```python
from build123d import *

# Parameters (mm, degrees)
SKETCH_1_R             = 6.25
SM_BASE_FLANGE_1_DEPTH = 6
OTHER_START            = 4.8
OTHER_1_OUTLINE_W      = 4.4
OTHER_1_OUTLINE_H      = 6
OTHER_1_DEPTH          = 20.4
OTHER_START_2          = 41.159902189
OTHER_1_2_OUTLINE_W    = 4.4
OTHER_1_2_OUTLINE_H    = 6
OTHER_1_2_DEPTH        = 20.4
OTHER_START_3          = 77.519804378
OTHER_1_3_OUTLINE_W    = 4.4
OTHER_1_3_OUTLINE_H    = 6
OTHER_1_3_DEPTH        = 20.4


# Read off the part's stored shape, not the designer's step: Выступы и прорези-Прорезь1
# Sheet-metal steps are written as plain solids
with BuildPart() as part:
    # Sketch 1 → Базовая кромка1 (new body)
    with BuildSketch(Plane.XY):
        with BuildLine():
            Line((0, 0), (0, -23))
            Line((0, -23), (92.230562732, -113.222677357))
            ThreePointArc((92.230562732, -113.222677357), (113.643192103, -112.780058395), (112.786839702, -91.379982025))
            ThreePointArc((112.786839702, -91.379982025), (92.360596545, -22.078545096), (144.700960487, 27.725138224))
            ThreePointArc((144.700960487, 27.725138224), (156.538037696, 42.016473572), (145.424946819, 56.877761338))
            ThreePointArc((145.424946819, 56.877761338), (102.719804378, 62.5), (60.014661936, 56.877761338))
            ThreePointArc((60.014661936, 56.877761338), (56.414969483, 55.389643277), (53.319804477, 53.024852653))
            Line((53.319804477, 53.024852653), (0, 0))
        make_face()
        with Locations((102.719804378, -102.5)):
            Circle(SKETCH_1_R, mode=Mode.SUBTRACT)
        with Locations((141.542661143, 42.388873943)):
            Circle(SKETCH_1_R, mode=Mode.SUBTRACT)
        with Locations((122.298733211, 46.216729206)):
            Circle(SKETCH_1_R, mode=Mode.SUBTRACT)
        with Locations((102.719804378, 47.5)):
            Circle(SKETCH_1_R, mode=Mode.SUBTRACT)
        with Locations((83.140875544, 46.216729206)):
            Circle(SKETCH_1_R, mode=Mode.SUBTRACT)
        with Locations((63.896947612, 42.388873943)):
            Circle(SKETCH_1_R, mode=Mode.SUBTRACT)
    extrude(amount=SM_BASE_FLANGE_1_DEPTH)

    # Other 1 outline → Other 1 (cut)
    with BuildSketch(Plane.YZ.offset(OTHER_START)):
        with Locations((-2, 3)):
            Rectangle(OTHER_1_OUTLINE_W, OTHER_1_OUTLINE_H)
    other_1 = extrude(amount=OTHER_1_DEPTH, mode=Mode.SUBTRACT)

    # Other 1 2 outline → Other 1 2 (cut)
    with BuildSketch(Plane.YZ.offset(OTHER_START_2)):
        with Locations((-2, 3)):
            Rectangle(OTHER_1_2_OUTLINE_W, OTHER_1_2_OUTLINE_H)
    other_1_2 = extrude(amount=OTHER_1_2_DEPTH, mode=Mode.SUBTRACT)

    # Other 1 3 outline → Other 1 3 (cut)
    with BuildSketch(Plane.YZ.offset(OTHER_START_3)):
        with Locations((-2, 3)):
            Rectangle(OTHER_1_3_OUTLINE_W, OTHER_1_3_OUTLINE_H)
    other_1_3 = extrude(amount=OTHER_1_3_DEPTH, mode=Mode.SUBTRACT)

    # Зеркальное отражение1: Other 1, Other 1 2, Other 1 3 across plane
    add(other_1.mirror(Plane.ZX.offset(-11.5)), mode=Mode.SUBTRACT)
    add(other_1_2.mirror(Plane.ZX.offset(-11.5)), mode=Mode.SUBTRACT)
    add(other_1_3.mirror(Plane.ZX.offset(-11.5)), mode=Mode.SUBTRACT)


solid = part.part
```
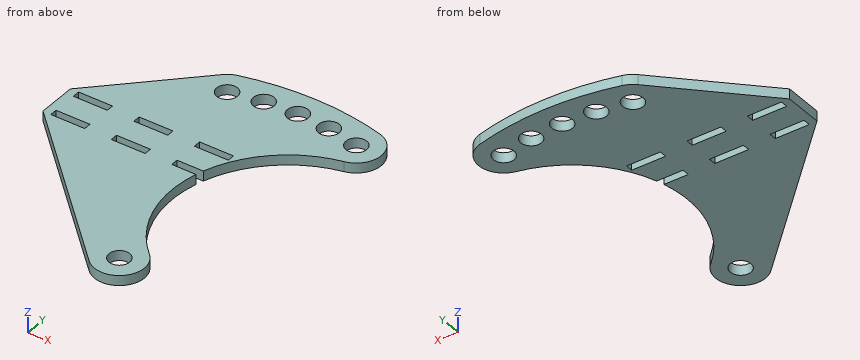
Here's how the part is built. I have some questions about the finished solid (model axes, mm). Give positions to 0.01 mm unless a question says otherwise; leave off trailing zeros. Write each loop counter-clockwise with the first axis right and the second up, starting at its lowest first coordinate (ties: lowest second). Pieces come first, ordered by that corner, then holes. Notation, with made-up numbers: M 88.25,8.25 L 125.25,8.25 A26 ccw 125.25,36.25 Z; hole C 50,14 d6. An arc over 180 degrees is marked long. Put each result on its own line as item: value. Start each with the question number.
Item 1: Will these pins go through, and if not, where does the flat tip stop? pin 1 (1.3 mm diameter, centred on y = -2.5, z = 2.5, fed in from -X); pin 2 (7.5 mm diameter, centred on x = 83.14, y = 46.22, fed in from +Z); pin 3 (1.8 mm diameter, centred on x = 47.5, z = 3.5, fed in from -Y); pin 4 (3 mm diameter, centred on x = 17.5, z = 2.5, fed in from -Y).
Item 2: If we section it at B-B, the plane y = -102.5: Write out the boundary of the cut face in (x, z), then the cut area to 3 significant figures.
Item 3: I need wall thicknesses on L1, parallel to X at y = -23, z = 2.65; L2, parallel to X at y = 43, z = 4.1; L3, parallel to Y at x = 100.5, z = 5.65. Which ranges of each line are inside material? Lowest first, please. Write a range as from..to.
Item 4: If we section it at D-D, the plane y = -13: Write out the boundary of the cut face in (x, z), then the cut area to 3 significant figures.
Item 5: If we section it at A-A, the plane x = 80: Write out the boundary of the cut face in (y, z).
Item 6: If we section it at C-C, the plane z = 4.05: Count the separate pieces of the cut face and the enclosed holes in it, then the cut area to 3 significant figures.
Values:
1. pin 1: x = 0
1. pin 2: through
1. pin 3: y = -70.35
1. pin 4: y = -41.59
2. outline: M 81.27,0 L 96.47,0 L 96.47,6 L 81.27,6 Z; M 108.97,0 L 117.72,0 L 117.72,6 L 108.97,6 Z
2. area: 144 mm²
3. L1: 0..4.8, 25.2..41.16, 61.56..77.52
3. L2: 43.24..57.68, 70.12..77.78, 88.5..98.38, 107.06..116.94, 127.66..135.32, 147.76..156.53
3. L3: -117.33..-108.34, -96.66..-76.69, -3.34..41.66, 53.34..62.49
4. outline: M 0,0 L 95.48,0 L 95.48,6 L 0,6 Z
4. area: 573 mm²
5. outline: M -101.26,0 L -23.2,0 L -23.2,6 L -101.26,6 Z; M -18.8,0 L -4.2,0 L -4.2,6 L -18.8,6 Z; M 0.2,0 L 40.81,0 L 40.81,6 L 0.2,6 Z; M 51.62,0 L 60.93,0 L 60.93,6 L 51.62,6 Z
6. separate pieces: 1
6. enclosed holes: 11
6. area: 12,400 mm²
